The model under review builds one solid part; all positions refer to its coordinate system, in mm. A direction names the side the tool comes from. Coordinates: 2 decimals unless noted, no trailing zeros. Order: outer loops, then holes, each group sorted by start corner. A loop starts at its lowest first (then second) coordinate and runs counter-clockwise, first axis right, second up.
```python
from build123d import *

# Parameters (mm, degrees)
CUT_EXTRUDE_1_DEPTH      = 1
SKETCH_3_R               = 6
EXTRUDE_1_DEPTH          = 6
SKETCH_4_R               = 3
EXTRUDE_2_DEPTH          = 15
SKETCH_5_W               = 8.431927353
SKETCH_5_H               = 1.818650998
CUT_EXTRUDE_2_DEPTH      = 12
SKETCH_6_R               = 1.5
CUT_EXTRUDE_3_DEPTH      = 5
SKETCH_8_R               = 2
CUT_EXTRUDE_4_DEPTH      = 5
CUT_EXTRUDE_5_DEPTH      = 74.793631162
CUT_EXTRUDE_5_DEPTH_BACK = 74.793631162
EXTRUDE_3_DEPTH          = 12
EXTRUDE_3_DEPTH_BACK     = 12
SKETCH_11_R              = 4.5
EXTRUDE_4_DEPTH          = 3
EXTRUDE_START            = 1.5
SKETCH_12_R              = 17.5
EXTRUDE_5_DEPTH          = 1.5
SKETCH_13_W              = 0.2
SKETCH_13_H              = 4
EXTRUDE_6_DEPTH          = 5
SKETCH_14_R              = 1.5
EXTRUDE_7_DEPTH          = 1
SKETCH_15_R              = 7
EXTRUDE_8_DEPTH          = 3.5
SKETCH_16_R              = 1.5
EXTRUDE_9_DEPTH          = 2


with BuildPart() as part:
    # Sketch 1 → Revolve 1 (revolve)
    with BuildSketch(Plane(origin=(0, 0, 0), x_dir=(1, 0, 0), z_dir=(0, 1, 0)), mode=Mode.PRIVATE) as revolve_1_sk:
        Polygon((0, 0), (0, 18.5), (19, 18.5), (19, 16.970676932), (22.5, 16.970676932), (22.5, 18), (48.5, 18), (48.5, 17.5), (69, 17.5), (69, 0), align=None)
    revolve(revolve_1_sk.sketch.rotate(Axis((-22.922421057, 0, 0), (1, 0, 0)), 180), axis=Axis((-22.922421057, 0, 0), (1, 0, 0)))

    # Sketch 2 → Cut-Extrude 1 (cut)
    with BuildSketch(Plane.ZY):
        with BuildLine():
            ThreePointArc((-8.94427191, 8), (0, -12), (8.94427191, 8))
            ThreePointArc((8.94427191, 8), (0, -2), (-8.94427191, 8))
        make_face()
    extrude(amount=-CUT_EXTRUDE_1_DEPTH, mode=Mode.SUBTRACT)

    # Sketch 3 → Extrude 1 (add)
    with BuildSketch(Plane.ZY):
        with Locations(Location((0, 7, 0), (0, 0, 180))):
            Circle(SKETCH_3_R)
    extrude(amount=EXTRUDE_1_DEPTH)

    # Sketch 4 → Extrude 2 (add)
    with BuildSketch(Plane.ZY.offset(6)):
        with Locations((0, 7)):
            Circle(SKETCH_4_R)
    extrude(amount=EXTRUDE_2_DEPTH)

    # Sketch 5 → Cut-Extrude 2 (cut)
    with BuildSketch(Plane.ZY.offset(21)):
        with Locations((0.29013852, 10.309325499)):
            Rectangle(SKETCH_5_W, SKETCH_5_H)
    extrude(amount=-CUT_EXTRUDE_2_DEPTH, mode=Mode.SUBTRACT)

    # Sketch 6 → Cut-Extrude 3 (cut)
    with BuildSketch(Plane.ZY):
        with Locations((-15.5, 0)):
            Circle(SKETCH_6_R)
        with Locations((-7.75, 13.423393759)):
            Circle(SKETCH_6_R)
        with Locations((7.75, 13.423393759)):
            Circle(SKETCH_6_R)
        with Locations((15.5, 0)):
            Circle(SKETCH_6_R)
        with Locations((7.75, -13.423393759)):
            Circle(SKETCH_6_R)
        with Locations((-7.75, -13.423393759)):
            Circle(SKETCH_6_R)
        with Locations((-13.423393759, 7.75)):
            Circle(SKETCH_6_R)
    extrude(amount=-CUT_EXTRUDE_3_DEPTH, mode=Mode.SUBTRACT)

    # Sketch 8 → Cut-Extrude 4 (cut)
    with BuildSketch(Plane.ZY):
        with Locations((-13.423393759, 7.75)):
            Circle(SKETCH_8_R)
        with Locations((13.423393759, 7.75)):
            Circle(SKETCH_8_R)
        with Locations((0, -15.5)):
            Circle(SKETCH_8_R)
    extrude(amount=-CUT_EXTRUDE_4_DEPTH, mode=Mode.SUBTRACT)

    # Sketch 9 → Cut-Extrude 5 (cut, two sides: drawn at the far end of the back side and taken through both)
    with BuildSketch(Plane.XY.offset(-CUT_EXTRUDE_5_DEPTH_BACK)):
        with BuildLine():
            Line((50.5, -6), (50.5, 6))
            ThreePointArc((50.5, 6), (53.5, 9), (56.5, 6))
            Line((56.5, 6), (56.5, -6))
            ThreePointArc((56.5, -6), (53.5, -9), (50.5, -6))
        make_face()
    extrude(amount=CUT_EXTRUDE_5_DEPTH + CUT_EXTRUDE_5_DEPTH_BACK, mode=Mode.SUBTRACT)

    # Sketch 10 → Extrude 3 (add, two sides: drawn at the far end of the back side and taken through both)
    with BuildSketch(Plane.XY.offset(-EXTRUDE_3_DEPTH_BACK)):
        with BuildLine():
            Line((50.5, 6), (50.5, -6))
            ThreePointArc((50.5, -6), (53.5, -9), (56.5, -6))
            Line((56.5, -6), (56.5, 6))
            ThreePointArc((56.5, 6), (53.5, 9), (50.5, 6))
        make_face()
    extrude(amount=EXTRUDE_3_DEPTH + EXTRUDE_3_DEPTH_BACK)

    # Sketch 11 → Extrude 4 (add)
    with BuildSketch(Plane(origin=(69, 0, 0), x_dir=(0, 0, -1), z_dir=(1, 0, 0))):
        with Locations(Location((0, 0, 0), (0, 0, 180))):
            Circle(SKETCH_11_R)
    extrude(amount=EXTRUDE_4_DEPTH)

    # Sketch 12 → Extrude 5 (add)
    with BuildSketch(Plane(origin=(72, 0, 0), x_dir=(0, 0, -1), z_dir=(1, 0, 0)).offset(EXTRUDE_START)):
        with Locations(Location((0, 0, 0), (0, 0, 180))):
            Circle(SKETCH_12_R)
    extrude(amount=-EXTRUDE_5_DEPTH)

    # Sketch 13 → Extrude 6 (add)
    with BuildSketch(Plane(origin=(73.5, 0, 0), x_dir=(0, 0, -1), z_dir=(1, 0, 0))):
        with Locations((-12.869137114, 0)):
            Rectangle(SKETCH_13_W, SKETCH_13_H)
        with Locations((12.869137114, 0)):
            Rectangle(SKETCH_13_W, SKETCH_13_H)
    extrude(amount=-EXTRUDE_6_DEPTH)

    # Sketch 14 → Extrude 7 (add)
    with BuildSketch(Plane(origin=(73.5, 0, 0), x_dir=(0, 0, -1), z_dir=(1, 0, 0))):
        Circle(SKETCH_14_R)
    extrude(amount=EXTRUDE_7_DEPTH)

    # Sketch 15 → Extrude 8 (add)
    with BuildSketch(Plane(origin=(74.5, 0, 0), x_dir=(0, 0, -1), z_dir=(1, 0, 0))):
        Circle(SKETCH_15_R)
    extrude(amount=EXTRUDE_8_DEPTH)

    # Sketch 16 → Extrude 9 (add)
    with BuildSketch(Plane(origin=(78, 0, 0), x_dir=(0, 0, -1), z_dir=(1, 0, 0))):
        Circle(SKETCH_16_R)
    extrude(amount=EXTRUDE_9_DEPTH)


solid = part.part
```
(1) We need section B-B, the plane y = -10. Write out the cut boundary in (x, z), and give its area (3 significant figures).
A:
outline: (0, -15.56) - (19, -15.56) - (19, -13.71) - (22.5, -13.71) - (22.5, -14.97) - (48.5, -14.97) - (48.5, -14.36) - (69, -14.36) - (69, 14.36) - (48.5, 14.36) - (48.5, 14.97) - (22.5, 14.97) - (22.5, 13.71) - (19, 13.71) - (19, 15.56) - (0, 15.56) - (0, 6.63) - (1, 6.63) - (1, -6.63) - (0, -6.63) - close; (72, -14.36) - (73.5, -14.36) - (73.5, 14.36) - (72, 14.36) - close
area: 2,080 mm2
(2) We need section D-D, the plane x = 53.5. Write out the cut boundary in (y, z), and give its area (3 significant figures).
A:
outline: (-9, -15.01) - (-9, -12) - (9, -12) - (9, -15.01) arc R17.5 ccw to (9, 15.01) - (9, 12) - (-9, 12) - (-9, 15.01) arc R17.5 ccw to start
area: 793 mm2
(3) Draft analysis for pull direction X (two halves, no side actions). For faces 4 (the face through (80, 0, 0)), 5 (the face through (70.48, -3.04, -3.32)), 6 (the face through (19, 16.4, 5.4)), 7 (the face through (-13.4, 4.07, -0.65)), state which applies: released by +X, released by -X, zero draft, split by the parting line, or undercut.
A:
face 4: released by +X
face 5: undercut
face 6: undercut
face 7: zero draft
(4) For pin 1 Ø10 at (x, z) = (11.5, 1) entering from +Y; pin 2 Ø2.5 at (y, z) = (-14, -7.5) entering from -X; pin 3 Ø4.5 at (y, z) = (-2, 13.5) entering from +X; pin 4 Ø15.5 at (y, z) = (2.5, 2) entering from +X, all flat-tipped, find the tip position at first contact; note any pin that passes through.
A:
pin 1: stops at y = 18.5
pin 2: stops at x = 0
pin 3: stops at x = 73.5
pin 4: stops at x = 80
(5) We need section C-C, the plane x = -11. Write out the cut boundary in (y, z).
A:
outline: (9.4, -1.8) - (9.4, 1.8) arc R3 ccw (long way) to start
(6) We need section A-A, the plane z = 10.5. Write out the cut boundary in (x, y), and give its area (3 significant figures).
A:
outline: (0, -15.23) - (19, -15.23) - (19, -13.33) - (22.5, -13.33) - (22.5, -14.62) - (48.5, -14.62) - (48.5, -14) - (69, -14) - (69, 14) - (48.5, 14) - (48.5, 14.62) - (22.5, 14.62) - (22.5, 13.33) - (19, 13.33) - (19, 15.23) - (0, 15.23) - (0, 5.81) - (1, 5.81) - (1, -5.81) - (0, -5.81) - close; (72, -14) - (73.5, -14) - (73.5, 14) - (72, 14) - close
area: 2,040 mm2
(7) Wall thickness on probe 1 along X at (y, z) = (-1, -16); probe 2 along Y at (x, z) = (0.7, 0); probe 3 along X at (y, z) = (-4, 5): over which ranges is each line inside the solid? List them lowest first.
A:
probe 1: x = 5 to 50.5, 56.5 to 69, 72 to 73.5
probe 2: y = -18.5 to -17.5, -13.5 to -12, -2 to 18.5
probe 3: x = 1 to 69, 72 to 73.5, 74.5 to 78
(8) Machinability: for faces 1 (the face through (71, 0, -12.769)), 2 (the face through (-15, 9.4, 0)), 3 (the face through (2, 0, 14)), which of the approach directions +Z, -Z, +X, -X, +Y, -Y give a long, thin tool a straight path to every point of the face, cutting with its end or side? Answer none if there is none.
A:
face 1: +Y, -Y
face 2: +Z, -Z, -X, +Y
face 3: -X
